The listing builds one solid part. Answer for the finished solid, in the listing's coordinates (mm). A direction names the side the tool comes from. Give positions to 0.01 mm unless a question says otherwise; leave off trailing zeros. Order: outer loops, then holes, each group sorted by start corner. A loop starts at its lowest first (then second) coordinate and runs counter-clockwise, first axis right, second up. Notation, with made-up numbers: (14, -26) - (45, -26) arc R14 ccw to (45, -10) - close; hole circle Ø9 at (11, 3.5). An arc over 180 degrees is marked (long way). Use a Markdown table: item, result. Add a question column.
1) Find section B-B, the plane x = 18. Determine the outline of the cut face in (y, z).
2) Flat-ended cylindrical pins translate along their axes: pin 1 (3 mm diameter, centred on x = 50, y = 35.5, fed in from -Z); pin 2 (10 mm diameter, centred on x = 27, y = 10, fed in from -Z); pin 3 (21.5 mm diameter, centred on y = 15.5, z = 491.5, fed in from -X); pin 4 (4 mm diameter, centred on x = 78, y = 9, fed in from +Z). Find the tip coordinate at first contact, or state that the pin passes through.
3) For faces 4 (the face through (23.68, -2.03, 601.07)), 5 (the face through (88.9, 15, 601)), 6 (the face through (28.59, 11.42, -12.52)), 7 (the face through (34, 21, 1216.66)), 8 (the face through (31.82, 2.45, 1232.08)), determine the directions among +Z, -Z, +X, -X, +Y, -Y from which every point of the face is accessible in a straight line to the end or side of a thin tool.
4) Straight lines are drawn through the part: line 1 (Z direction, x = 75.5, y = 8); line 2 (X direction, y = 22.5, z = 608); line 3 (X direction, y = 28, z = 1009.5). For each, find the intervals that lie inside material, in ascending order.
5) Find section A-A, the plane z = 817.5. Determine the outline of the cut face in (x, y).
6) The mould has two halves that part along X. Classify faces 1 (the face through (0, 14, 601)), 2 (the face through (44, 36.83, 601)), 3 (the face through (2.54, 16, 601)): released by +X, released by -X, zero draft, split by the parting line, or undercut.
from build123d import *

# Parameters (mm, degrees)
BOSS_EXTRUDE1_DEPTH    = 1219.2
SKETCH2_W              = 1219.2
SKETCH2_H              = 7.62
BOSS_EXTRUDE2_DEPTH    = 2.54
SKETCH3_W              = 1219.2
SKETCH3_H              = 7.62
BOSS_EXTRUDE3_DEPTH    = 2.54
SKETCH4_R              = 15.875
SKETCH4_R_2            = 12.7
BOSS_EXTRUDE4_DEPTH    = 25.4
BOSS_EXTRUDE5_START    = 25.4
SKETCH6_R              = 15.875
SKETCH6_R_2            = 12.7
BOSS_EXTRUDE5_DEPTH    = 25.4
SHELL2_START           = 2.54
SHELL2_DEPTH           = 1214.12
SKETCH9_W              = 93.98
SKETCH9_H              = 1219.2
BOSS_EXTRUDE7_DEPTH    = 2.54
FILLET1_R              = 2.54
CUT_EXTRUDE3_START     = -2.54
CUT_EXTRUDE3_OUTLINE_R = 12.7
CUT_EXTRUDE3_DEPTH     = 2.54
SKETCH11_R             = 12.7
CUT_EXTRUDE4_DEPTH     = 2.54
CUT_EXTRUDE5_REACH     = 1250.616
SKETCH12_W             = 25.4
SKETCH12_H             = 25.4
LPATTERN1_COUNT        = 6
LPATTERN1_PITCH        = 203.2


# Read off the part's stored shape, not the designer's step: Shell2, Cut-Extrude3
with BuildPart() as part:
    # Sketch1 → Boss-Extrude1 (new body)
    with BuildSketch(Plane.XY):
        Polygon((0, 0), (0, 34.29), (88.9, 34.29), (88.9, 0), (44.45, -3.81), align=None)
    extrude(amount=BOSS_EXTRUDE1_DEPTH)

    # Sketch2 → Boss-Extrude2 (add)
    with BuildSketch(Plane(origin=(88.9, 0, 0), x_dir=(0, 0, -1), z_dir=(1, 0, 0))):
        with Locations((-609.6, 30.48)):
            Rectangle(SKETCH2_W, SKETCH2_H)
    extrude(amount=BOSS_EXTRUDE2_DEPTH)

    # Sketch3 → Boss-Extrude3 (add)
    with BuildSketch(Plane.ZY):
        with Locations((609.6, 30.48)):
            Rectangle(SKETCH3_W, SKETCH3_H)
    extrude(amount=BOSS_EXTRUDE3_DEPTH)

    # Sketch4 → Boss-Extrude4 (add)
    with BuildSketch(Plane(origin=(0, 0, 0), x_dir=(-1, 0, 0), z_dir=(0, 0, -1))):
        with Locations(Location((-44.45, 12.065, 0), (0, 0, 260.201815092))):
            Circle(SKETCH4_R)
        with Locations((-44.45, 12.065)):
            Circle(SKETCH4_R_2, mode=Mode.SUBTRACT)
    extrude(amount=BOSS_EXTRUDE4_DEPTH)

    # Sketch6 → Boss-Extrude5 (add)
    with BuildSketch(Plane.XY.offset(1219.2).offset(BOSS_EXTRUDE5_START)):
        with Locations(Location((44.45, 12.065, 0), (0, 0, 279.798184908))):
            Circle(SKETCH6_R)
        with Locations(Location((44.45, 12.065, 0), (0, 0, 180))):
            Circle(SKETCH6_R_2, mode=Mode.SUBTRACT)
    extrude(amount=-BOSS_EXTRUDE5_DEPTH)

    # Shell2 outline → Shell2 (cut)
    with BuildSketch(Plane.XY.offset(SHELL2_START)):
        Polygon((44.45, -1.260686463), (86.36, 2.331599251), (86.36, 29.21), (88.9, 29.21), (88.9, 34.29), (0, 34.29), (0, 29.21), (2.54, 29.21), (2.54, 2.331599251), align=None)
    extrude(amount=SHELL2_DEPTH, mode=Mode.SUBTRACT)

    # Sketch9 → Boss-Extrude7 (add)
    with BuildSketch(Plane(origin=(0, 34.29, 0), x_dir=(1, 0, 0), z_dir=(0, 1, 0))):
        with Locations((44.45, -609.6)):
            Rectangle(SKETCH9_W, SKETCH9_H)
    extrude(amount=BOSS_EXTRUDE7_DEPTH)

    # Fillet1
    fillet1_edges = [part.edges().sort_by_distance(p)[0] for p in [
        (0, 0, 609.6),
        (88.9, 0, 609.6),
    ]]
    fillet(fillet1_edges, radius=FILLET1_R)

    # Cut-Extrude3 outline → Cut-Extrude3 (cut)
    with BuildSketch(Plane(origin=(0, 0, 0), x_dir=(-1, 0, 0), z_dir=(0, 0, -1)).offset(CUT_EXTRUDE3_START)):
        with Locations((-44.45, 12.065)):
            Circle(CUT_EXTRUDE3_OUTLINE_R)
    extrude(amount=CUT_EXTRUDE3_DEPTH, mode=Mode.SUBTRACT)

    # Sketch11 → Cut-Extrude4 (cut)
    with BuildSketch(Plane.XY.offset(1219.2)):
        with Locations((44.45, 12.065)):
            Circle(SKETCH11_R)
    extrude(amount=-CUT_EXTRUDE4_DEPTH, mode=Mode.SUBTRACT)

    # Sketch12 → Cut-Extrude5 (cut, up to next)
    with BuildSketch(Plane(origin=(0, 36.83, 0), x_dir=(1, 0, 0), z_dir=(0, 1, 0)), mode=Mode.PRIVATE) as cut_extrude5_sk1:
        with Locations((44.45, -1155.7)):
            Rectangle(SKETCH12_W, SKETCH12_H)
    cut_extrude5_tool1 = extrude(cut_extrude5_sk1.sketch, amount=-CUT_EXTRUDE5_REACH, mode=Mode.PRIVATE) & part.part
    cut_extrude5 = cut_extrude5_tool1.solids().sort_by_distance((44.45, 36.83, 1155.7))[0]
    add(cut_extrude5, mode=Mode.SUBTRACT)

    # LPattern1: Cut-Extrude5 ×6
    with Locations(*[(0, 0, -i * LPATTERN1_PITCH) for i in range(1, LPATTERN1_COUNT)]):
        add(cut_extrude5, mode=Mode.SUBTRACT)


solid = part.part
The answers:
| question | item | result |
|---|---|---|
| 1 | outline | (-1.54, 0) - (36.83, 0) - (36.83, 1219.2) - (-1.54, 1219.2) - close; hole (1.01, 2.54) - (34.29, 2.54) - (34.29, 1216.66) - (1.01, 1216.66) - close |
| 2 | pin 1 | z = 0 |
| 2 | pin 2 | z = -25.4 |
| 2 | pin 3 | x = 0 |
| 2 | pin 4 | z = 1219.2 |
| 3 | face 4 | +Z, -Z, -X, -Y |
| 3 | face 5 | +Z, -Z, +X, -Y |
| 3 | face 6 | -Z |
| 3 | face 7 | none |
| 3 | face 8 | +Z |
| 4 | line 1 | 0 to 2.54, 1216.66 to 1219.2 |
| 4 | line 2 | 0 to 2.54, 86.36 to 88.9 |
| 4 | line 3 | -2.54 to 2.54, 86.36 to 91.44 |
| 5 | outline | (-2.54, 26.67) - (0, 26.67) - (0, 2.33) arc R2.54 ccw to (2.32, -0.2) - (44.45, -3.81) - (86.58, -0.2) arc R2.54 ccw to (88.9, 2.33) - (88.9, 26.67) - (91.44, 26.67) - (91.44, 36.83) - (-2.54, 36.83) - close; hole (0, 29.21) - (2.54, 29.21) - (2.54, 2.33) - (44.45, -1.26) - (86.36, 2.33) - (86.36, 29.21) - (88.9, 29.21) - (88.9, 34.29) - (0, 34.29) - close |
| 6 | face 1 | released by -X |
| 6 | face 2 | zero draft |
| 6 | face 3 | undercut |
